Geometry: see drawing. Coordinates: mm, zero at the bounding-box minimum. A direction names the side the tool comes from. Coordinates: 2 decimals unless noted, no trailing zeros. Write each loop counter-clockwise with the first axis right and the second up, starting at its lowest first coordinate (ties: lowest second). Pieces come first, ordered by that corner, then holes. Notation, with made-up numbers: (38.25, -19.5) - (60.25, -19.5) arc R21 cw to (60.25, 1.5) - close; hole circle Ø11 at (37, 15). An arc over 180 degrees is marked (long way). Use CSV: the item, a comma, the result in double quotes.
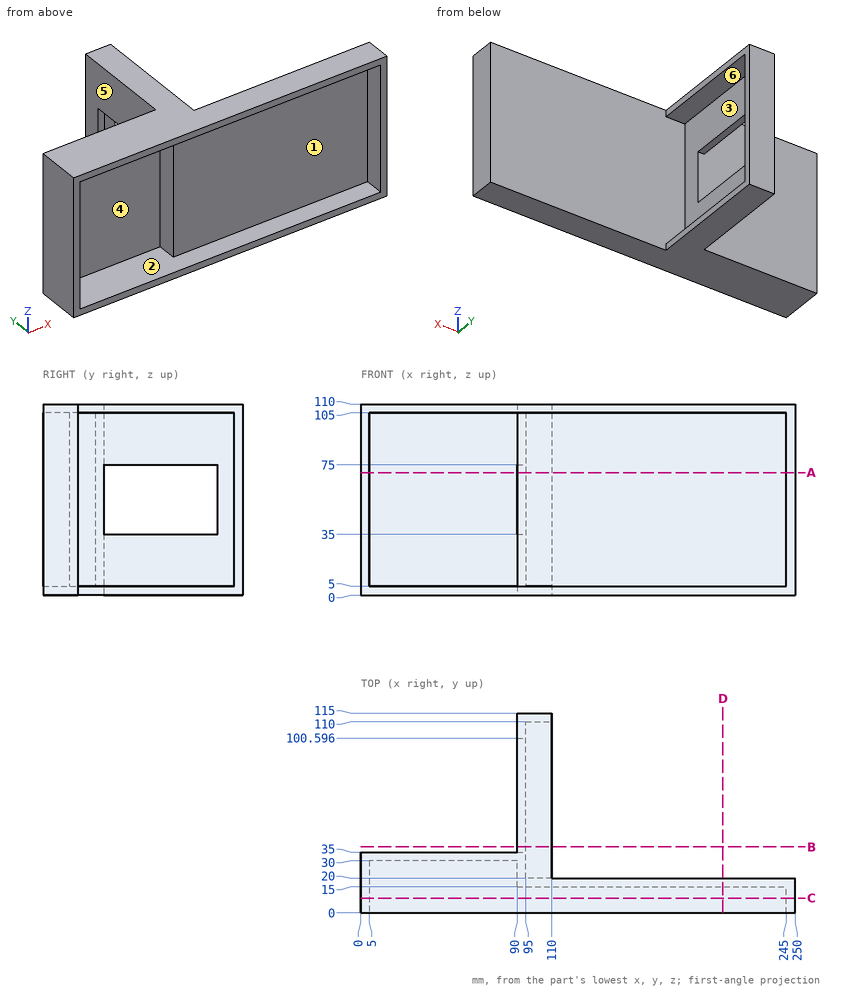
(1) Ray query, probe 1 along Z at (x, y) = (43.5, 28.5); probe 2 along X at (y, z) = (51.5, 105.5); probe 3 along X at (y, z) = (32, 61.5). Return the intervals inside material, ascending. Write a range as from..to.
Check values:
probe 1,"0..5, 105..110"
probe 2,"90..110"
probe 3,"0..95"
(2) Cut plane D-D on x = 208.5. Return loops of the section in (y, z).
Check values:
outline,"(0, 0) - (20, 0) - (20, 110) - (0, 110) - (0, 105) - (15, 105) - (15, 5) - (0, 5) - close"
(3) Draft query along Y for the marked faces 1, 2 and 3. Return one class per face: pulls with the +Y half, pulls with the -Y half, needs draft (parallel to the pull), parting line crosses it, or undercut.
Check values:
face 1,"pulls with the -Y half"
face 2,"needs draft"
face 3,"undercut"
(4) Cut plane C-C on y = 8.5. Return loops of the section in (x, z), and give its area (3 significant figures).
Check values:
outline,"(0, 0) - (250, 0) - (250, 110) - (0, 110) - close; hole (5, 5) - (245, 5) - (245, 105) - (5, 105) - close"
area,"3,500 mm^2"
(5) Cut plane A-A on z = 70.5. Return loops of the section in (x, y), and give its area (3 significant figures).
Check values:
outline,"(0, 0) - (5, 0) - (5, 30) - (90, 30) - (90, 15) - (245, 15) - (245, 0) - (250, 0) - (250, 20) - (95, 20) - (95, 35) - (0, 35) - close; (90, 100.6) - (95, 100.6) - (95, 110) - (110, 110) - (110, 115) - (90, 115) - close"
area,"1,700 mm^2"
(6) Pin query (flat end, axial travel): pin 1 Ø1.5 at (x, z) = (87, 94.5) entering from +Y; pin 2 Ø4 at (y, z) = (91, 22.5) entering from +X; pin 3 Ø12 at (x, z) = (196.5, 62) entering from -Y; pin 4 Ø1 at (y, z) = (100, 45.5) entering from -X. Return the tip coordinate at first contact, or that it passes through.
Check values:
pin 1,"y = 35"
pin 2,"x = 95"
pin 3,"y = 15"
pin 4,"through"
(7) Cut plane B-B on y = 38. Return loops of the section in (x, z), and give its area (3 significant figures).
Check values:
outline,"(90, 0) - (110, 0) - (110, 5) - (95, 5) - (95, 35) - (90, 35) - close; (90, 75) - (95, 75) - (95, 105) - (110, 105) - (110, 110) - (90, 110) - close"
area,"500 mm^2"
(8) Reachability of the marked faces 4, 5 and 6 from +Z, -Z, +X, -X, +Y, -Y: full face, straight path, thin tool, end or side. Return the list, or none.
Check values:
face 4,"-Y"
face 5,"+Z, -Z, -X, +Y"
face 6,"+X"
